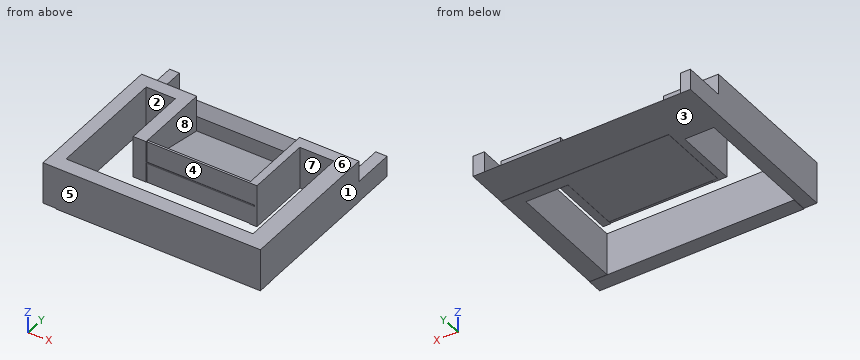
from build123d import *

# Parameters (mm, degrees)
F0_W      = 7.9096108675
F0_H      = 89.265525341
F1_DEPTH  = 25.4
F2_W      = 9.0597718954
F2_H      = 25.8198998213
F3_DEPTH  = 123.5302612185
F4_W      = 10.519862175
F4_H      = 25.5959949732
F5_DEPTH  = 80.2284926176
F6_W      = 6.8411193788
F6_H      = 25.5959949732
F7_DEPTH  = 25.4
F8_W      = 7.6834112406
F8_H      = 25.4
F9_DEPTH  = 25.4
F10_W     = 4.7150052428
F10_H     = 25.7374218941
F11_DEPTH = 38.8002488762
F12_W     = 1.2486185879
F12_H     = 25.4
F13_DEPTH = 61.9014054537
F14_W     = 7.7484271765
F14_H     = 25.4
F15_DEPTH = 38.1346493959
F16_W     = 44.0207533538
F16_H     = 3.7513971329
F17_DEPTH = 65.4726680368
F19_DEPTH = 65.2894191444
F20_W     = 5.9870034456
F20_H     = 12.7
F21_DEPTH = 25.4
F23_DEPTH = 118.6141502112
F24_W     = 6.8387184292
F24_H     = 12.6020025134
F25_DEPTH = 25.4


with BuildPart() as f1:
    # F0 (on Top) → F1 (new body)
    with BuildSketch(Plane.XY):
        with Locations((-61.7658346891, -0.2627521753)):
            Rectangle(F0_W, F0_H)
    extrude(amount=F1_DEPTH)

    # F2 (on face) → F3 (join)
    with BuildSketch(Plane.YZ.offset(-57.8110292554)):
        with Locations((-40.3656288981, 12.4900500894)):
            Rectangle(F2_W, F2_H)
    extrude(amount=F3_DEPTH)

    # F4 (on face) → F5 (join)
    with BuildSketch(Plane(origin=(0, -35.8357429504, 0), x_dir=(-1, 0, 0), z_dir=(0, 1, 0))):
        with Locations((-60.4593008757, 12.6020025134)):
            Rectangle(F4_W, F4_H)
    extrude(amount=F5_DEPTH)

    # F6 (on face) → F7 (join)
    with BuildSketch(Plane(origin=(55.1993697882, 0, 0), x_dir=(0, -1, 0), z_dir=(-1, 0, 0))):
        with Locations((-40.9721899778, 12.6020025134)):
            Rectangle(F6_W, F6_H)
    extrude(amount=F7_DEPTH)

    # F8 (on face) → F9 (join)
    with BuildSketch(Plane.YZ.offset(-57.8110292554)):
        with Locations((40.5283048749, 12.7)):
            Rectangle(F8_W, F8_H)
    extrude(amount=F9_DEPTH)

    # F10 (on face) → F11 (join)
    with BuildSketch(Plane.XZ.offset(-37.5516302884)):
        with Locations((32.1568724096, 12.531289053)):
            Rectangle(F10_W, F10_H)
    extrude(amount=F11_DEPTH)

    # F12 (on face) → F13 (join)
    with BuildSketch(Plane(origin=(29.7993697882, 0, 0), x_dir=(0, -1, 0), z_dir=(-1, 0, 0))):
        with Locations((0.6243092939, 12.7)):
            Rectangle(F12_W, F12_H)
    extrude(amount=F13_DEPTH)

    # F14 (on face) → F15 (join)
    with BuildSketch(Plane.XZ.offset(-36.6865992546)):
        with Locations((-36.2852428436, 12.7)):
            Rectangle(F14_W, F14_H)
    extrude(amount=F15_DEPTH)

    # F16 (on face) → F17 (join)
    with BuildSketch(Plane(origin=(29.7993697882, 0, 0), x_dir=(0, -1, 0), z_dir=(-1, 0, 0))):
        with Locations((-22.3823729903, 1.6797035933)):
            Rectangle(F16_W, F16_H)
    extrude(amount=F17_DEPTH)

    # F18 (on face) → F19 (join)
    with BuildSketch(Plane.YZ.offset(-32.4110292554)):
        Polygon((44.3700104952, 3.5554021597), (-1.4480501413, 12.7), (0.3719963133, 3.5554021597), align=None)
    extrude(amount=F19_DEPTH)

    # F20 (on face) → F21 (join)
    with BuildSketch(Plane(origin=(0, 44.3700104952, 0), x_dir=(-1, 0, 0), z_dir=(0, 1, 0))):
        with Locations((62.7271384001, 6.35)):
            Rectangle(F20_W, F20_H)
    extrude(amount=F21_DEPTH)

    # F22 (on face) → F23 (join)
    with BuildSketch(Plane.YZ.offset(-59.7336366773)):
        Polygon((69.7700104952, 0), (44.3700104952, 12.7), (44.3700104952, 0), align=None)
    extrude(amount=F23_DEPTH)

    # F24 (on face) → F25 (join)
    with BuildSketch(Plane(origin=(0, 44.3927496672, 0), x_dir=(-1, 0, 0), z_dir=(0, 1, 0))):
        with Locations((-62.2998727486, 6.3010012567)):
            Rectangle(F24_W, F24_H)
    extrude(amount=F25_DEPTH)


solid = f1.part
Model file for the job. Use its own axes, mm. Face numbers are marked on the shaded views. A direction names the side the tool comes from. Round coordinates to 2 decimals unless told otherwise and drop trailing zeros. Loops run counter-clockwise (first coordinate to the right, second up) from the corner with the lowest first, then second, coordinate; pieces in that order, holes last. Notation, with made-up numbers: (88, -20.75) - (111, -20.75) arc R15 ccw to (111, -8.75) - close; hole circle Ø3 at (69.25, 0). An arc over 180 degrees is marked (long way). Write each question's results on one line, items separated by ' | '.
(1) Saw through at A-A, the plane y = -27.5. List the corners of the cut face in (x, z), then the cut area to 3 significant figures.
Answer below:
outline: (-65.72, 0) - (-57.81, 0) - (-57.81, 25.4) - (-65.72, 25.4) - close; (55.2, -0.2) - (65.72, -0.2) - (65.72, 25.4) - (55.2, 25.4) - close | area: 470 mm^2
(2) Saw through at C-C, the plane z = 23.25. List the corners of the cut face in (x, y), then the cut area to 3 significant figures.
Answer below:
outline: (-65.72, -44.9) - (65.72, -44.9) - (65.72, 44.39) - (29.8, 44.39) - (29.8, 0) - (-32.1, 0) - (-32.1, -1.25) - (34.51, -1.25) - (34.51, 37.55) - (55.2, 37.55) - (55.2, -35.84) - (-57.81, -35.84) - (-57.81, 36.69) - (-40.16, 36.69) - (-40.16, -1.45) - (-32.41, -1.45) - (-32.41, 44.37) - (-65.72, 44.37) - close | area: 3,590 mm^2
(3) Pin check, flat tips, straight feed: pin 1 (5.5 mm diameter, centred on x = 63.5, y = 59.5, fed in from +Z); pin 2 (10 mm diameter, centred on x = 24.5, y = 41, fed in from +Z); pin 3 (14.5 mm diameter, centred on x = -16, z = 21, fed in from +Y). Stop position of each tip, or through.
Answer below:
pin 1: stops at z = 12.6 | pin 2: stops at z = 12.7 | pin 3: stops at y = 0
(4) 3-axis set-ups, long thin cutter, end or side, ignore diameter. For the marked faces 4, 5, 6, 7 and 8: which of +Z, -Z, +X, -X, +Y, -Y reach the whole face in a straight line?
Answer below:
face 4: none | face 5: +Z, -Z, +X, -X, -Y | face 6: +Z, +X, -X, +Y, -Y | face 7: +Z, -Z | face 8: +Z
(5) Wall check: L1, parallel to X at y = 27.5, z = 19.5; L2, parallel to Y at x = 53, z = 15.5; L3, parallel to X at y = -3.5, z = 21. Give the ranges that are in metal, low to high.
Answer below:
L1: x = -65.72 to -57.81, -40.16 to -32.41, 29.8 to 34.51, 55.2 to 65.72 | L2: y = -44.9 to -35.84, 37.55 to 44.39 | L3: x = -65.72 to -57.81, 55.2 to 65.72
(6) Mould opens along X. For the marked faces 1, 2 and 3 say: released by +X, released by -X, zero draft, split by the parting line, or undercut.
Answer below:
face 1: released by +X | face 2: undercut | face 3: zero draft
(7) Saw through at B-B, the plane x = -43.5. List the corners of the cut face in (y, z), then the cut area to 3 significant figures.
Answer below:
outline: (-44.9, -0.42) - (-35.84, -0.42) - (-35.84, 25.4) - (-44.9, 25.4) - close; (36.69, 0) - (69.77, 0) - (44.37, 12.7) - (44.37, 25.4) - (36.69, 25.4) - close | area: 590 mm^2
(8) Saw through at D-D, the plane y = 31. List the corners of the cut face in (x, z), then the cut area to 3 significant figures.
Answer below:
outline: (-65.72, 0) - (-57.81, 0) - (-57.81, 25.4) - (-65.72, 25.4) - close; (-40.16, 0) - (-35.67, 0) - (-35.67, -0.2) - (29.8, -0.2) - (29.8, -0.34) - (34.51, -0.34) - (34.51, 25.4) - (29.8, 25.4) - (29.8, 6.22) - (-32.41, 6.22) - (-32.41, 25.4) - (-40.16, 25.4) - close; (55.2, -0.2) - (65.72, -0.2) - (65.72, 25.4) - (55.2, 25.4) - close | area: 1,190 mm^2
